```python
from build123d import *

# Parameters (mm, degrees)
ESQUISSE1_R        = 12.125
BOSS_EXTRU_1_DEPTH = 30.91
ESQUISSE2_R        = 3.2
BOSS_EXTRU_2_DEPTH = 1.1
ESQUISSE3_R        = 1
BOSS_EXTRU_3_DEPTH = 13.54
ESQUISSE9_W        = 1.7
ESQUISSE9_H        = 1.7
BOSS_EXTRU_6_DEPTH = 2.6


with BuildPart() as part:
    # Esquisse1 → Boss.-Extru.1 (new body)
    with BuildSketch(Plane.XY):
        with Locations(Location((0, 0, 0), (0, 0, 180))):
            Circle(ESQUISSE1_R)
    extrude(amount=BOSS_EXTRU_1_DEPTH)

    # Esquisse2 → Boss.-Extru.2 (add)
    with BuildSketch(Plane.XY.offset(30.91)):
        Circle(ESQUISSE2_R)
    extrude(amount=BOSS_EXTRU_2_DEPTH)

    # Esquisse3 → Boss.-Extru.3 (add)
    with BuildSketch(Plane.XY.offset(32.01)):
        Circle(ESQUISSE3_R)
    extrude(amount=BOSS_EXTRU_3_DEPTH)

    # Esquisse9 → Boss.-Extru.6 (add)
    with BuildSketch(Plane(origin=(0, 0, 0), x_dir=(-1, 0, 0), z_dir=(0, 0, -1))):
        with Locations((0, -9.275)):
            Rectangle(ESQUISSE9_W, ESQUISSE9_H)
        with Locations((0, 9.275)):
            Rectangle(ESQUISSE9_W, ESQUISSE9_H)
    extrude(amount=BOSS_EXTRU_6_DEPTH)


solid = part.part
```
Model file for the job. Use its own axes, mm. A direction names the side the tool comes from. Round coordinates to 2 decimals unless told otherwise and drop trailing zeros. Write each loop counter-clockwise with the first axis right and the second up, starting at its lowest first coordinate (ties: lowest second). Pieces come first, ordered by that corner, then holes. Notation, with made-up numbers: (11.5, 36) - (24.5, 36) arc R26 cw to (24.5, 64) - close; hole circle Ø9 at (14.25, 50.25). An arc over 180 degrees is marked (long way). Use CSV: the item, a comma, the result in double quotes. Start each with the question number.
Item 1: Drill centre lines: L1, parallel to Z at x = -8.25, y = 5.25; L2, parallel to X at y = 10, z = 14.5; L3, parallel to Z at x = 0, y = -8.5. Where is each one in solid material? Low to high. Write a range as [from, to].
Item 2: Band-saw the part on C-C (z = 15). Write the cut outline in (x, y) (3 decimals).
Item 3: Band-saw the part on B-B (x = 0). Write the cut outline in (y, z) (3 decimals), and give its area (3 significant figures).
Item 4: Two-plate mould, pull along Y, no slides. Class faces 5 (the face through (0, -8.425, -1)), 6 (the face through (0.85, -9, -1)), 7 (the face through (0, -1, 39)), 8 (the face through (0, 8.425, -1)): released by +Y, released by -Y, zero draft, split by the parting line, or undercut.
Item 5: Band-saw the part on A-A (y = 0). Write the cut outline in (x, z) (3 decimals), and give its area (3 significant figures).
Item 6: Pin check, flat tips, straight feed: P1, Ø6, axis at x = -3.5, y = 7.5, coming from the +Z side; P2, Ø0.8, axis at y = -9.5, z = -1, coming from the +X side; P3, Ø1.4, axis at x = -0.5, z = -2, coming from the +Y side (3 decimals). Stop position of each tip, or through.
Item 7: Tool access for faces 1 (the face through (-3, 3, 30.91)), 2 (the face through (0, -10.125, -1)), 3 (the face through (0, 10.125, -1)), 4 (the face through (0.85, 9, -1)): list every direction of +Z, -Z, +X, -X, +Y, -Y with a clear straight run to the whole face (end or side of a thin tool).
Item 8: Band-saw the part on D-D (z = 32.5). Write the cut outline in (x, y).
Checked values:
1,L1,"z = [0, 30.91]"
1,L2,"x = [-6.86, 6.86]"
1,L3,"z = [-2.6, 30.91]"
2,outline,"circle Ø24.25 at (0, 0)"
3,outline,"(-12.125, 0) - (-10.125, 0) - (-10.125, -2.6) - (-8.425, -2.6) - (-8.425, 0) - (8.425, 0) - (8.425, -2.6) - (10.125, -2.6) - (10.125, 0) - (12.125, 0) - (12.125, 30.91) - (3.2, 30.91) - (3.2, 32.01) - (1, 32.01) - (1, 45.55) - (-1, 45.55) - (-1, 32.01) - (-3.2, 32.01) - (-3.2, 30.91) - (-12.125, 30.91) - close"
3,area,"793 mm²"
4,face 5,"undercut"
4,face 6,"zero draft"
4,face 7,"split by the parting line"
4,face 8,"undercut"
5,outline,"(-12.125, 0) - (12.125, 0) - (12.125, 30.91) - (3.2, 30.91) - (3.2, 32.01) - (1, 32.01) - (1, 45.55) - (-1, 45.55) - (-1, 32.01) - (-3.2, 32.01) - (-3.2, 30.91) - (-12.125, 30.91) - close"
5,area,"784 mm²"
6,P1,"stops at z = 30.91"
6,P2,"stops at x = 0.85"
6,P3,"stops at y = 10.125"
7,face 1,"+Z"
7,face 2,"-Z, +X, -X, -Y"
7,face 3,"-Z, +X, -X, +Y"
7,face 4,"-Z, +X, +Y, -Y"
8,outline,"circle Ø2 at (0, 0)"
